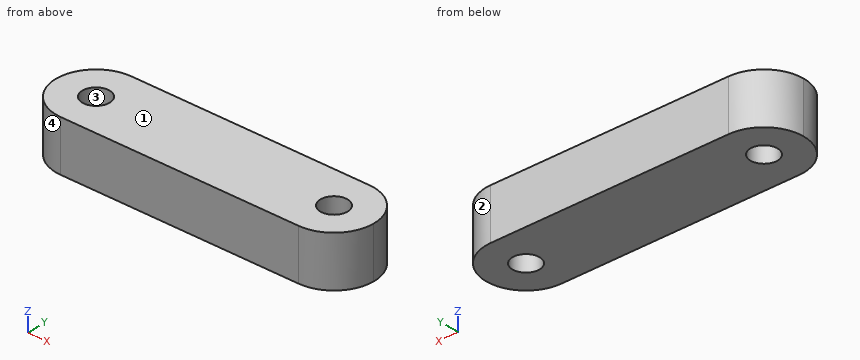
```python
from build123d import *

# Parameters (mm, degrees)
SKETCH1_W           = 40
SKETCH1_H           = 10
SKETCH1_R           = 1.7
BOSS_EXTRUDE1_DEPTH = 6.35
FILLET1_R           = 5


with BuildPart() as part:
    # Sketch1 → Boss-Extrude1 (new body)
    with BuildSketch(Plane.XY):
        with Locations((20, 5)):
            Rectangle(SKETCH1_W, SKETCH1_H)
        with Locations((35, 5)):
            Circle(SKETCH1_R, mode=Mode.SUBTRACT)
        with Locations((5, 5)):
            Circle(SKETCH1_R, mode=Mode.SUBTRACT)
    extrude(amount=BOSS_EXTRUDE1_DEPTH)

    # Fillet1
    fillet1_edges = [part.edges().sort_by_distance(p)[0] for p in [
        (0, 10, 3.175),
        (0, 0, 3.175),
        (40, 10, 3.175),
        (40, 0, 3.175),
    ]]
    fillet(fillet1_edges, radius=FILLET1_R - 0.0001)  # a hair under: the kernel refuses the full size


solid = part.part
```
The listing builds one solid part. Answer for the finished solid, in the listing's coordinates (mm). Face numbers are marked on the shaded views. Coordinates: 2 decimals unless noted, no trailing zeros. Write each loop counter-clockwise with the first axis right and the second up, starting at its lowest first coordinate (ties: lowest second). Pieces come first, ordered by that corner, then holes. Notation, with made-up numbers: (-24, 22) - (-9, 22) arc R21 ccw to (-9, 52) - close; hole circle Ø9 at (87.5, 44.5). An arc over 180 degrees is marked (long way). Return JSON: item names as keys, results as strings. Group by question number.
Q1. Find the intervals of material crossed by line 1 along X through (y, z) = (4, 1); line 2 along Y through (x, z) = (35, 3.5); line 3 along X through (y, z) = (3.75, 4.5), in increasing order. Write a range as [from, to].
Q2. The part is cut by section A-A on z = 1.75. State how many separate pieces and enclosed holes the cut face has, and give its area (3 significant figures).
Q3. The part is cut by section D-D on y = 9.5. Write down the section's boundary in (x, z).
Q4. The part is cut by section C-C on y = 2.25. Write down the section's boundary in (x, z), and give its area (3 significant figures).
Q5. For a pull along X with two mould halves and no side action, classify the marked faces 1, 2, 3 and 4 as +X half, -X half, draft (parallel to the pull), parting line (faces both ways), or undercut.
Q6. The part is cut by section B-B on y = 6.25. Write down the section's boundary in (x, z), and give its area (3 significant figures).
Q7. A flat-ended cylindrical pin translates along its axis: pin 1 Ø1.5 at (y, z) = (8, 4.5) entering from +X. Find the tip coordinate at first contact, or state that the pin passes through.
Evaluation:
{
 "1": {"line 1": "x = [0.1, 3.63], [6.37, 33.63], [36.37, 39.9]", "line 2": "y = [0, 3.3], [6.7, 10]", "line 3": "x = [0.16, 3.85], [6.15, 33.85], [36.15, 39.84]"},
 "2": {"separate pieces": "1", "enclosed holes": "2", "area": "360 mm2"},
 "3": {"outline": "(2.82, 0) - (37.18, 0) - (37.18, 6.35) - (2.82, 6.35) - close"},
 "4": {"outline": "(0.82, 0) - (39.18, 0) - (39.18, 6.35) - (0.82, 6.35) - close", "area": "244 mm2"},
 "5": {"face 1": "draft", "face 2": "+X half", "face 3": "undercut", "face 4": "-X half"},
 "6": {"outline": "(0.16, 0) - (3.85, 0) - (3.85, 6.35) - (0.16, 6.35) - close; (6.15, 0) - (33.85, 0) - (33.85, 6.35) - (6.15, 6.35) - close; (36.15, 0) - (39.84, 0) - (39.84, 6.35) - (36.15, 6.35) - close", "area": "223 mm2"},
 "7": {"pin 1": "stops at x = 39.47"}
}
